Here's how the part is built. I have some questions about the finished solid (model axes, mm). A direction names the side the tool comes from. Coordinates: 2 decimals unless noted, no trailing zeros. Write each loop counter-clockwise with the first axis right and the second up, starting at its lowest first coordinate (ties: lowest second). Pieces come first, ordered by that corner, then holes. Notation, with made-up numbers: M 23,44 L 48,44 A18 cw 48,58 Z; hole C 14,12.25 d8. An arc over 180 degrees is marked long. Use a Markdown table: item, result.
```python
from build123d import *

# Parameters (mm, degrees)
BOSS_EXTRUDE1_DEPTH = 82.55


with BuildPart() as part:
    # Sketch1 → Boss-Extrude1 (new body)
    with BuildSketch(Plane.XY):
        with BuildLine():
            Line((174.498, 0), (-6.477, 0))
            Line((-6.477, 0), (-6.477, -143.1925))
            ThreePointArc((-6.477, -143.1925), (-6.012032015, -144.315032015), (-4.8895, -144.78))
            Line((-4.8895, -144.78), (172.9105, -144.78))
            ThreePointArc((172.9105, -144.78), (174.033032015, -144.315032015), (174.498, -143.1925))
            Line((174.498, -143.1925), (174.498, 0))
        make_face()
        with BuildLine():
            Line((6.223, -114.3), (22.225, -114.3))
            ThreePointArc((22.225, -114.3), (24.47006403, -115.22993597), (25.4, -117.475))
            Line((25.4, -117.475), (25.4, -132.08))
            Line((25.4, -132.08), (142.621, -132.08))
            Line((142.621, -132.08), (142.621, -117.475))
            ThreePointArc((142.621, -117.475), (143.55093597, -115.22993597), (145.796, -114.3))
            Line((145.796, -114.3), (161.798, -114.3))
            Line((161.798, -114.3), (161.798, -30.48))
            Line((161.798, -30.48), (145.796, -30.48))
            ThreePointArc((145.796, -30.48), (143.55093597, -29.55006403), (142.621, -27.305))
            Line((142.621, -27.305), (142.621, -12.7))
            Line((142.621, -12.7), (25.4, -12.7))
            Line((25.4, -12.7), (25.4, -27.305))
            ThreePointArc((25.4, -27.305), (24.47006403, -29.55006403), (22.225, -30.48))
            Line((22.225, -30.48), (6.223, -30.48))
            Line((6.223, -30.48), (6.223, -114.3))
        make_face(mode=Mode.SUBTRACT)
    extrude(amount=BOSS_EXTRUDE1_DEPTH)


solid = part.part
```
1. Suppose I cut it at A-A on x = 43. Write out the boundary of the cut face in (y, z).
Answers follow:
| item | result |
|---|---|
| outline | M -144.78,0 L -132.08,0 L -132.08,82.55 L -144.78,82.55 Z; M -12.7,0 L 0,0 L 0,82.55 L -12.7,82.55 Z |
2. We'd pull the mould along X, two halves only. Please class faces 3 (the face through (-6.477, -71, 41)), 4 (the face through (83, -7, 82.55)), 5 (the face through (25.4, -125, 41)): +X half, -X half, draft (parallel to the pull), parting line (faces both ways), or undercut.
Answers follow:
| item | result |
|---|---|
| face 3 | -X half |
| face 4 | draft |
| face 5 | undercut |
3. Which directions (+Z, -Z, +X, -X, +Y, -Y) give clear straight access to the entire face, cutting with the end or side of a thin tool? Please do faces 1 (the face through (154, -114.3, 41)), 2 (the face through (85, 0, 41)).
Answers follow:
| item | result |
|---|---|
| face 1 | +Z, -Z |
| face 2 | +Z, -Z, +X, -X, +Y |
4. Suppose I cut it at B-B on y = -101.5. Write out the boundary of the cut face in (x, z), and give its area (3 significant figures).
Answers follow:
| item | result |
|---|---|
| outline | M -6.48,0 L 6.22,0 L 6.22,82.55 L -6.48,82.55 Z; M 161.8,0 L 174.5,0 L 174.5,82.55 L 161.8,82.55 Z |
| area | 2,100 mm2 |
5. I need wall thicknesses on probe 1 along X at (y, z) = (-59, 39.5); probe 2 along Y at (x, z) = (69, 39); probe 3 along X at (y, z) = (-119.5, 63.5). Which ranges of each line are inside material? Lowest first, please.
Answers follow:
| item | result |
|---|---|
| probe 1 | x = -6.48 to 6.22, 161.8 to 174.5 |
| probe 2 | y = -144.78 to -132.08, -12.7 to 0 |
| probe 3 | x = -6.48 to 25.4, 142.62 to 174.5 |
